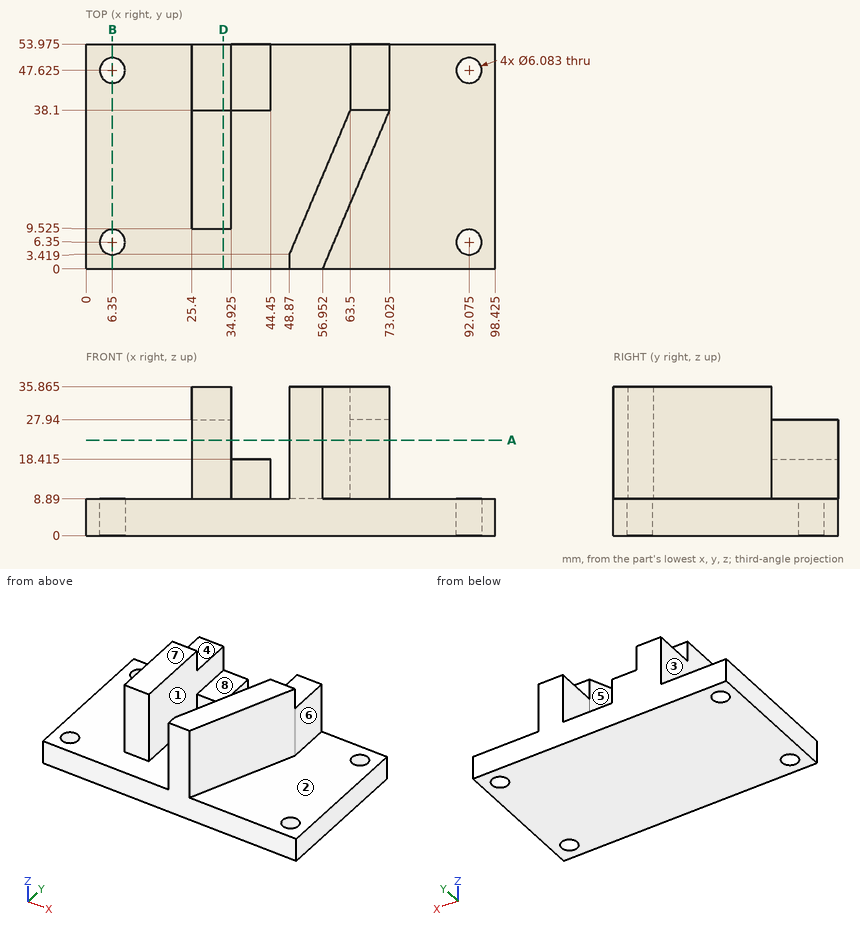
Can you work these out from the drawing? Everything is in mm from the part's minimum corner. A direction names the side the tool comes from. Round coordinates to 2 decimals unless told otherwise and drop trailing zeros. Order: outer loops, then holes, each group sorted by start corner. A loop starts at its lowest first (then second) coordinate and runs counter-clockwise, first axis right, second up. Notation, with made-up numbers: (-26, -27.75) - (30, -27.75) arc R13 cw to (30, -2.75) - close; hole circle Ø4 at (-16.5, -24). An arc over 180 degrees is marked (long way). Answer in a Markdown table with one row per item.
(1) Suppose I cut it at B-B, the plane x = 6.35. Please give me the cut outline in (y, z) (1 decimal), plus the area to 3 significant figures.
From the geometry:
| item | result |
|---|---|
| outline | (0, 0) - (3.3, 0) - (3.3, 8.9) - (0, 8.9) - close; (9.4, 0) - (44.6, 0) - (44.6, 8.9) - (9.4, 8.9) - close; (50.7, 0) - (54, 0) - (54, 8.9) - (50.7, 8.9) - close |
| area | 372 mm2 |
(2) Suppose I cut it at D-D, the plane x = 33. Please give me the cut outline in (y, z) (1 decimal), plus the area to 3 significant figures.
From the geometry:
| item | result |
|---|---|
| outline | (0, 0) - (54, 0) - (54, 27.9) - (38.1, 27.9) - (38.1, 35.9) - (9.5, 35.9) - (9.5, 8.9) - (0, 8.9) - close |
| area | 1,550 mm2 |
(3) Please list where these lines run through material, in increasing order: L1, parallel to X at y = 6, z = 2 (1 decimal); L2, parallel to X at y = 49, z = 7 (1 decimal); L3, parallel to Z at x = 89, y = 41. Write a range as from..to.
From the geometry:
| item | result |
|---|---|
| L1 | x = 0..3.3, 9.4..89.1, 95.1..98.4 |
| L2 | x = 0..3.6, 9.1..89.4, 94.8..98.4 |
| L3 | z = 0..8.89 |
(4) For P1, Ø7, axis at x = 92.075, y = 6.35, coming from the -Z side; P2, Ø3, axis at x = 31, z = 21, coming from the -Y side (3 decimals); P3, Ø10, axis at y = 7.5, z = 16.5, coming from the -X side; P4, Ø3.5, axis at x = 6.35, y = 47.625, coming from the +Z side, each with a flat end and sliding along its axis, tell me the tip position at first contact or that it passes through.
From the geometry:
| item | result |
|---|---|
| P1 | stops at z = 0 |
| P2 | stops at y = 9.525 |
| P3 | stops at x = 25.4 |
| P4 | passes through |
(5) Which directions (+Z, -Z, +X, -X, +Y, -Y) give clear straight access to the entire face, cutting with the end or side of a thin tool? Please do the marked faces 1, 2, 3, 4 and 5.
From the geometry:
| item | result |
|---|---|
| face 1 | +Z, -Y |
| face 2 | +Z, +X, -Y |
| face 3 | +Z, -X, +Y, -Y |
| face 4 | +Z, +X, -X, +Y |
| face 5 | +Z, +Y |
(6) Suppose I cut it at A-A, the plane z = 23. Please give me the cut outline in (x, y) (1 decimal).
From the geometry:
| item | result |
|---|---|
| outline | (25.4, 9.5) - (34.9, 9.5) - (34.9, 54) - (25.4, 54) - close; (48.9, 0) - (57, 0) - (73, 38.1) - (73, 54) - (63.5, 54) - (63.5, 38.1) - (48.9, 3.4) - close |
(7) If we mould it in two halves opening along X, with no side actions, what happens to the marked faces 6, 7 and 8? For each: released by +X, released by -X, zero draft, split by the parting line, or undercut.
From the geometry:
| item | result |
|---|---|
| face 6 | released by +X |
| face 7 | zero draft |
| face 8 | undercut |
